Geometry: see drawing. Coordinates: mm, zero at the bounding-box minimum. Round coordinates to 2 decimals unless told otherwise and drop trailing zeros. Loops run counter-clockwise (first coordinate to the right, second up) from the corner with the lowest first, then second, coordinate; pieces in that order, holes last.
(1) Material intervals for probe 1 along Y at (x, z) = (18, 7.25) (1 decimal); probe 2 along Y at (x, z) = (17.5, 3); probe 3 along X at (y, z) = (4.5, 9.25) (1 decimal), sorted ascending.
(2) Mould query, pull axis X, two halves, no side actions, for the marked faces 1 and 2. Classes: pulls with the +X half, pulls with the -X half, needs draft (parallel to the pull), parting line crosses it, or undercut.
(3) First-contact query: pin 1 Ø1 at (y, z) = (11, 4.5) entering from +X; pin 2 Ø1.5 at (y, z) = (19.5, 8) entering from -X; pin 3 Ø3 at (y, z) = (14, 8.5) entering from -X. Flat tips, straight axial feed; report the tip coordinate or a pass-through.
(4) Section C-C, the plane z = 5.5. Return the cut outline in (x, y).
(5) Section D-D, the plane z = 11.25. Return the cut outline in (x, y).
(6) Section A-A, the plane x = 18. Return the cut outline in (y, z).
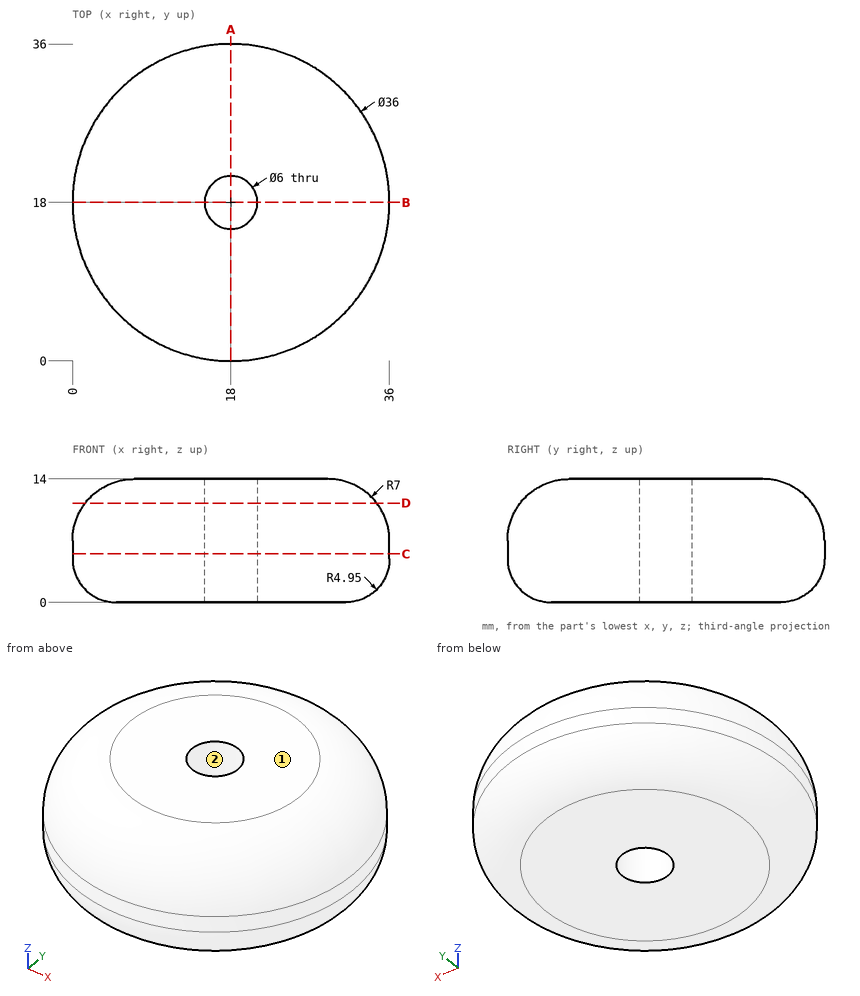
Output values:
1. probe 1: y = 0 to 15, 21 to 36
1. probe 2: y = 0.41 to 15.04, 20.96 to 35.59
1. probe 3: x = 6.7 to 29.3
2. face 1: needs draft
2. face 2: undercut
3. pin 1: stops at x = 34.77
3. pin 2: stops at x = 0.04
3. pin 3: stops at x = 0.24
4. outline: circle Ø36 at (18, 18); hole circle Ø6 at (18, 18)
5. outline: circle Ø33.12 at (18, 18); hole circle Ø6 at (18, 18)
6. outline: (0, 4.95) arc R4.95 ccw to (4.95, 0) - (15, 0) - (15, 14) - (7, 14) arc R7 ccw to (0, 7) - close; (21, 0) - (31.05, 0) arc R4.95 ccw to (36, 4.95) - (36, 7) arc R7 ccw to (29, 14) - (21, 14) - close
